from build123d import *

# Parameters (mm, degrees)
F2_SIZE = 2
F3_SIZE = 0.5


with BuildPart() as f1:
    # F0 (on Front) → F1 (revolve)
    with BuildSketch(Plane.XZ):
        Polygon((0, 32), (0, 0), (13.5, 0), (13.5, 15), (5.5, 15), (5.5, 20), (2.5, 20), (2.5, 32), align=None)
    revolve(axis=Axis((0, 0, 16), (0, 0, -1)))

    # F2
    f2_edges = [f1.edges().sort_by_distance(p)[0] for p in [
        (-13.5, 0, 15),
        (-13.5, 0, 0),
    ]]
    chamfer(f2_edges, length=F2_SIZE)

    # F3
    f3_edges = [f1.edges().sort_by_distance(p)[0] for p in [
        (-2.5, 0, 32),
    ]]
    chamfer(f3_edges, length=F3_SIZE)


solid = f1.part
Source: CAD feature listing. Evaluate the final solid. Frame: model axes, mm. A direction names the side the tool comes from. Coordinates: 2 decimals unless noted, no trailing zeros. Loops run counter-clockwise (first coordinate to the right, second up) from the corner with the lowest first, then second, coordinate; pieces in that order, holes last. Notation, with made-up numbers: (-23.5, 16) - (20.5, 16) arc R27 cw to (20.5, 33) - close; hole circle Ø7 at (56, 6.5). An arc over 180 degrees is marked (long way). One line per question, with ' | ' between items.
1) First-contact query: P1, Ø2, axis at x = -5.5, z = 4.5, coming from the -Y side; P2, Ø5, axis at y = 2.5, z = 16.5, coming from the +X side; P3, Ø1.5, axis at y = 6, z = 8, coming from the -X side; P4, Ø4, axis at x = -1.5, y = -3, coming from the +Z side. Flat tips, straight axial feed; report the tip coordinate or a pass-through.
Report:
P1: stops at y = -12.73 | P2: stops at x = 12.29 | P3: stops at x = -12.44 | P4: stops at z = 32
2) Section A-A, the plane x = 0. Return loops of the section in (y, z).
Report:
outline: (-13.5, 2) - (-11.5, 0) - (11.5, 0) - (13.5, 2) - (13.5, 13) - (11.5, 15) - (5.5, 15) - (5.5, 20) - (2.5, 20) - (2.5, 31.5) - (2, 32) - (-2, 32) - (-2.5, 31.5) - (-2.5, 20) - (-5.5, 20) - (-5.5, 15) - (-11.5, 15) - (-13.5, 13) - close
3) Set-up query: faces 1 (the face through (5, -3, 15)), 2 (the face through (0, 0, 0)). Return all of +Z, -Z, +X, -X, +Y, -Y with unobstructed straight access to the full face (end or side cutting, diameter ignored); none if empty.
Report:
face 1: +Z | face 2: -Z, +X, -X, +Y, -Y
4) Section D-D, the plane z = 22. Return loops of the section in (x, y).
Report:
outline: circle Ø5 at (0, 0)
5) Line query: line 1 along Z through (x, y) = (5.5, 5.25); line 2 along X through (y, z) = (1.5, 30); line 3 along Y through (x, z) = (-3.75, 7). Output: solid intervals per line, ascending.
Report:
line 1: z = 0 to 15 | line 2: x = -2 to 2 | line 3: y = -12.97 to 12.97
6) Section C-C, the plane z = 7. Return loops of the section in (x, y).
Report:
outline: circle Ø27 at (0, 0)
